```python
from build123d import *

# Parameters (mm, degrees)
SKETCH1_W           = 127
SKETCH1_H           = 76.2
SKETCH1_R           = 6.35
BOSS_EXTRUDE1_DEPTH = 38.1
SKETCH3_W           = 38.1
SKETCH3_H           = 76.2
CUT_EXTRUDE1_DEPTH  = 25.4
FILLET1_R           = 12.7
CHAMFER1_SIZE       = 3.175
SHELL1_T            = -2.54


with BuildPart() as part:
    # Sketch1 → Boss-Extrude1 (new body)
    with BuildSketch(Plane.XY):
        Rectangle(SKETCH1_W, SKETCH1_H)
        with Locations((-44.45, 19.05)):
            Circle(SKETCH1_R, mode=Mode.SUBTRACT)
        with Locations((44.45, 19.05)):
            Circle(SKETCH1_R, mode=Mode.SUBTRACT)
        with Locations((-44.45, -19.05)):
            Circle(SKETCH1_R, mode=Mode.SUBTRACT)
        with Locations((44.45, -19.05)):
            Circle(SKETCH1_R, mode=Mode.SUBTRACT)
    extrude(amount=BOSS_EXTRUDE1_DEPTH)

    # Sketch3 → Cut-Extrude1 (cut)
    with BuildSketch(Plane.XY.offset(38.1)):
        Rectangle(SKETCH3_W, SKETCH3_H)
    extrude(amount=-CUT_EXTRUDE1_DEPTH, mode=Mode.SUBTRACT)

    # Fillet1
    fillet1_edges = [part.edges().sort_by_distance(p)[0] for p in [
        (63.5, -38.1, 19.05),
        (-63.5, -38.1, 19.05),
        (-63.5, 38.1, 19.05),
        (63.5, 38.1, 19.05),
    ]]
    fillet(fillet1_edges, radius=FILLET1_R)

    # Chamfer1
    chamfer1_edges = [part.edges().sort_by_distance(p)[0] for p in [
        (-50.8, 19.05, 38.1),
        (38.1, 19.05, 38.1),
        (-50.8, -19.05, 38.1),
        (38.1, -19.05, 38.1),
        (34.925, -38.1, 38.1),
        (-34.925, 38.1, 38.1),
        (19.05, 38.1, 25.4),
        (0, -38.1, 12.7),
        (19.05, -38.1, 25.4),
        (-19.05, -38.1, 25.4),
        (0, 38.1, 12.7),
        (-19.05, 38.1, 25.4),
        (-34.925, -38.1, 38.1),
        (-63.5, 0, 38.1),
        (-59.780256121, 34.380256121, 38.1),
        (-59.780256121, -34.380256121, 38.1),
        (63.5, 0, 38.1),
        (34.925, 38.1, 38.1),
        (59.780256121, 34.380256121, 38.1),
        (59.780256121, -34.380256121, 38.1),
    ]]
    chamfer(chamfer1_edges, length=CHAMFER1_SIZE)

    # Shell1
    shell1_openings = [part.faces().sort_by_distance(p)[0] for p in [
        (-50.8, -19.05, 0),
    ]]
    offset(amount=SHELL1_T, openings=shell1_openings, kind=Kind.INTERSECTION)


solid = part.part
```
The listing builds one solid part. Answer for the finished solid, in the listing's coordinates (mm). A direction names the side the tool comes from. Give positions to 0.01 mm unless a question says otherwise; leave off trailing zeros. Loops run counter-clockwise (first coordinate to the right, second up) from the corner with the lowest first, then second, coordinate; pieces in that order, holes last. Notation, with made-up numbers: (55, 48) - (104, 48) arc R16 ccw to (104, 63) - close; hole circle Ø3 at (52.5, 20). An arc over 180 degrees is marked (long way). Return JSON: item names as keys, results as strings. Group by question number.
1. Given pin 1 Ø8 at (x, y) = (-16, -3.5) entering from -Z; pin 2 Ø5 at (x, y) = (3.5, 2) entering from +Z, each flat-ended and moving along its own axis, determine where each tip first touches the part or whether it passes through.
2. Determine the mould class of faces 1 (the conical face through (57.183, 31.644, 35.103)), 2 (the conical face through (-58.093, -32.855, 37.196)), 3 (the conical face through (-58.255, 32.693, 37.196)), 4 (the cylindrical face through (57.905, -32.663, 17.174)) for opening direction Y: pulls with the +Y half, pulls with the -Y half, needs draft (parallel to the pull), parting line crosses it, or undercut.
3. Which of the six approach directions +Z, -Z, +X, -X, +Y, -Y give full straight-line access (tool end or side, diameter ignored) to faces 5 (the flat face through (20.615, 36.49, 24.013)), 6 (the flat face through (-41, 0, 35.56)), 7 (the flat face through (-19.05, 0, 26)), 8 (the flat face through (-34.703, -36.535, 36.49))?
4. Find section A-A (z = 32). State how many separate pieces and enclosed holes the cut face has, then the cut area to 3 significant figures.
5. Find section B-B (x = 6.5). Write down the section's boundary in (y, z) (3 decimals), then the cut area to 3 significant figures.
6. Straight lines are drawn through the part: line 1 (Y direction, x = 44, z = 10); line 2 (X direction, y = -1, z = 30.5); line 3 (X direction, y = -27, z = 15). For each, find the intervals that lie inside material, in ascending order. Write a range as [from, to].
Verdict:
{
 "1": {"pin 1": "stops at z = 10.16", "pin 2": "stops at z = 12.7"},
 "2": {"face 1": "undercut", "face 2": "pulls with the -Y half", "face 3": "pulls with the +Y half", "face 4": "undercut"},
 "3": {"face 5": "+Z, +Y", "face 6": "-Z", "face 7": "+Z, +Y, -Y", "face 8": "+Z, +X, -X, -Y"},
 "4": {"separate pieces": "6", "enclosed holes": "6", "area": "1,600 mm^2"},
 "5": {"outline": "(-38.1, 0) - (-35.56, 0) - (-35.56, 8.473) - (-33.873, 10.16) - (33.873, 10.16) - (35.56, 8.473) - (35.56, 0) - (38.1, 0) - (38.1, 9.525) - (34.925, 12.7) - (-34.925, 12.7) - (-38.1, 9.525) - close", "area": "238 mm^2"},
 "6": {"line 1": "y = [-38.1, -35.56], [-27.93, -25.38], [-12.72, -10.17], [10.17, 12.72], [25.38, 27.93], [35.56, 38.1]", "line 2": "x = [-63.5, -60.96], [-21.59, -19.05], [19.05, 21.59], [60.96, 63.5]", "line 3": "x = [-63.4, -60.83], [-48.43, -40.47], [-21.59, -19.05], [19.05, 21.59], [40.47, 48.43], [60.83, 63.4]"}
}
